Check sheet for the modelled part. Datum: model origin and axes. Units: mm. A direction names the side the tool comes from. Give positions to 0.01 mm unless a question says otherwise; leave off trailing zeros. Loops run counter-clockwise (first coordinate to the right, second up) from the corner with the lowest first, then second, coordinate; pieces in that order, holes last. Notation, with made-up numbers: M 25,72.5 L 81,72.5 A19 ccw 81,80.5 Z; hole C 39,44 d6. An arc over 180 degrees is marked long. One line per question, with ' | ' between items. Start each with the question number.
from build123d import *

# Parameters (mm, degrees)
SKETCH1_R           = 11.049
SKETCH1_R_2         = 1.6
SKETCH1_R_3         = 1.524
BOSS_EXTRUDE1_DEPTH = 3.175


with BuildPart() as part:
    # Sketch1 → Boss-Extrude1 (new body)
    with BuildSketch(Plane.XY):
        with BuildLine():
            Line((57.15, -17.99971), (63.5, -17.99971))
            Line((63.5, -17.99971), (63.5, 7.40029))
            ThreePointArc((63.5, 7.40029), (62.57006403, 9.64535403), (60.325, 10.57529))
            Line((60.325, 10.57529), (46.1645, 10.57529))
            Line((46.1645, 10.57529), (46.1645, 7.40029))
            Line((46.1645, 7.40029), (42.9895, 7.40029))
            Line((42.9895, 7.40029), (42.9895, 10.57529))
            add(Edge.make_bspline(
                [(12.727717, 12.727717), (15.734639389, 9.720794612), (35.054158727, 10.57529), (42.9895, 10.57529)],
                knots=[0, 0, 0, 0, 1, 1, 1, 1], degree=3))
            ThreePointArc((12.727717, 12.727717), (12.029263941, 13.389786), (11.296423453, 14.013578318))
            ThreePointArc((11.296423453, 14.013578318), (10.59915166, 14.89503307), (10.3505, 15.991081784))
            Line((10.3505, 15.991081784), (10.3505, 40.126055474))
            ThreePointArc((10.3505, 40.126055474), (0, 50.476555474), (-10.3505, 40.126055474))
            Line((-10.3505, 40.126055474), (-10.3505, 15.991081784))
            ThreePointArc((-10.3505, 15.991081784), (-10.59915166, 14.89503307), (-11.296423453, 14.013578318))
            ThreePointArc((-11.296423453, 14.013578318), (-16.973949244, -5.989541481), (0, -17.99971))
            Line((0, -17.99971), (28.829, -17.99971))
            Line((28.829, -17.99971), (28.829, -14.82471))
            Line((28.829, -14.82471), (35.179, -14.82471))
            Line((35.179, -14.82471), (35.179, -11.14171))
            Line((35.179, -11.14171), (33.528, -11.14171))
            Line((33.528, -11.14171), (33.528, -8.34771))
            Line((33.528, -8.34771), (39.878, -8.34771))
            Line((39.878, -8.34771), (39.878, -11.14171))
            Line((39.878, -11.14171), (38.227, -11.14171))
            Line((38.227, -11.14171), (38.227, -14.82471))
            Line((38.227, -14.82471), (50.927, -14.82471))
            Line((50.927, -14.82471), (50.927, -11.14171))
            Line((50.927, -11.14171), (49.276, -11.14171))
            Line((49.276, -11.14171), (49.276, -8.34771))
            Line((49.276, -8.34771), (55.626, -8.34771))
            Line((55.626, -8.34771), (55.626, -11.14171))
            Line((55.626, -11.14171), (53.975, -11.14171))
            Line((53.975, -11.14171), (53.975, -14.82471))
            Line((53.975, -14.82471), (57.15, -14.82471))
            Line((57.15, -14.82471), (57.15, -17.99971))
        make_face()
        Circle(SKETCH1_R, mode=Mode.SUBTRACT)
        with Locations((9.899834348, 9.899834348)):
            Circle(SKETCH1_R_2, mode=Mode.SUBTRACT)
        with Locations((9.899834348, -9.899834348)):
            Circle(SKETCH1_R_2, mode=Mode.SUBTRACT)
        with Locations((-9.899834348, -9.899834348)):
            Circle(SKETCH1_R_2, mode=Mode.SUBTRACT)
        with Locations((-9.899834348, 9.899834348)):
            Circle(SKETCH1_R_2, mode=Mode.SUBTRACT)
        with Locations((44.577, 0.41529)):
            Circle(SKETCH1_R_3, mode=Mode.SUBTRACT)
        with BuildLine():
            Line((4.0005, 40.126055474), (4.0005, 22.664731685))
            ThreePointArc((4.0005, 22.664731685), (0, 18.664231685), (-4.0005, 22.664731685))
            Line((-4.0005, 22.664731685), (-4.0005, 40.126055474))
            ThreePointArc((-4.0005, 40.126055474), (0, 44.126555474), (4.0005, 40.126055474))
        make_face(mode=Mode.SUBTRACT)
    extrude(amount=BOSS_EXTRUDE1_DEPTH)


solid = part.part
Q1. Draft check along Y on faces 1 (the flat face through (53, 10.575, 2)), 2 (the flat face through (56, -14.825, 2)), 3 (the cylindrical face through (-0.088, 44.126, 1.565)). Enter one of: released by +Y, released by -Y, zero draft, split by the parting line, or undercut.
Q2. Cross-section at A-A (y = 24.5). Record the cut outline in (x, z) (1 decimal), and give its area (3 significant figures).
Q3. Cross-section at C-C (y = 41.5). Record the cut outline in (x, z) (3 decimals).
Q4. Cross-section at B-B (z = 2.4). State how many separate pieces and enclosed holes the cut face has, and give its area (3 significant figures).
Q5. Depth check by flat-ended pin: P1, Ø1.6, axis at y = 28.5, z = 1.5, coming from the -X side; P2, Ø0.8, axis at x = 34.5, z = 1, coming from the +Y side; P3, Ø1.6, axis at y = 8.5, z = 1.5, coming from the +X side; P4, Ø2.5, axis at x = -9.9, y = 9.9, coming from the -Z side. Enter the tip coordinate at first touch or a pass-through.
Q6. Material ranges on probe 1 along Y at (x, z) = (0, 2.1); probe 2 along X at (y, z) = (40, 1.35); probe 3 along Y at (x, z) = (34, 1.55), recorded low to high. Write a range as from..to.
Q7. Access from +Z, -Z, +X, -X, +Y, -Y to the whole of each face (thin tool, end or side, straight path). Record for faces 4 (the flat face through (37, -8.348, 2)), 5 (the flat face through (10.35, 28, 2)), 6 (the flat face through (35.179, -13, 2)), 7 (the flat face through (45, 7.4, 2)).
Solved:
1) face 1: released by +Y | face 2: released by -Y | face 3: undercut
2) outline: M -10.4,0 L -4,0 L -4,3.2 L -10.4,3.2 Z; M 4,0 L 10.4,0 L 10.4,3.2 L 4,3.2 Z | area: 40.3 mm²
3) outline: M -10.259,0 L -3.757,0 L -3.757,3.175 L -10.259,3.175 Z; M 3.757,0 L 10.259,0 L 10.259,3.175 L 3.757,3.175 Z
4) separate pieces: 1 | enclosed holes: 7 | area: 2,280 mm²
5) P1: stops at x = -10.35 | P2: stops at y = 10.48 | P3: stops at x = 63.49 | P4: passes through
6) probe 1: y = -18..-11.05, 11.05..18.66, 44.13..50.48 | probe 2: x = -10.35..-4, 4..10.35 | probe 3: y = -14.82..-11.14, -8.35..10.48
7) face 4: +Z, -Z | face 5: +Z, -Z, +X, +Y | face 6: +Z, -Z, -Y | face 7: +Z, -Z, +Y
